Part model, mm, in its own coordinate system. Coordinates: 2 decimals unless noted, no trailing zeros. Write each loop counter-clockwise with the first axis right and the second up, starting at its lowest first coordinate (ties: lowest second). Pieces come first, ordered by that corner, then holes. Notation, with made-up numbers: (80.5, 25.25) -> (125.5, 25.25) arc R32 cw to (125.5, 60.25) -> close; hole circle Ø3 at (51, -16.75). An arc over 180 degrees is marked (long way). Write item = value, one per line.
Autodesk Inventor part; units mm, degrees
ref_plane "YZ Plane" through (0, 0, 0) normal (1, 0, 0) x (0, 1, 0)
ref_plane "XZ Plane" through (0, 0, 0) normal (0, 1, 0) x (-1, 0, 0)
ref_plane "XY Plane" through (0, 0, 0) normal (0, 0, 1) x (1, 0, 0)
sketch "スケッチ1" plane through (0, 0, 0) normal (0, 0, 1) x (1, 0, 0)
  circle A0 centre (-5, 0) radius 1.55
  line L0 (0, 0) -> (-5, 0) construction
  line L1 (0, 0) -> (5, 0) construction
  circle A1 centre (5, 0) radius 1.55
  line L2 (-5, 3) -> (5, 3)
  arc A2 (-5, 3) -> (-5, -3) centre (-5, 0) ccw
  line L3 (-5, -3) -> (5, -3)
  arc A3 (5, -3) -> (5, 3) centre (5, 0) ccw
  dimension "d0" = 5
  dimension "d1" = 3.1
  dimension "d2" = 3
extrude "押し出し1" add sketch "スケッチ1" along normal blind 8
properties part number "胴体_サブフレーム_1_8" material "アセタール樹脂、黒"
Q1. Probe line 1 (X direction, y = -0.5, z = 4.5); line 2 (Y direction, x = 5, z = 3.25); line 3 (X direction, y = 0.95, z = 4.5). List the from-to ranges inside material, lowest first. Write a range as from..to.
Model answer:
line_1 = -7.96..-6.47, -3.53..3.53, 6.47..7.96
line_2 = -3..-1.55, 1.55..3
line_3 = -7.85..-6.22, -3.78..3.78, 6.22..7.85
Q2. Mould opens along X. For faces 1 (the face through (0, 0, 8)), 2 (the face through (8, 0, 4)), 3 (the face through (3.45, -0.07, 3.94)) say: released by +X, released by -X, zero draft, split by the parting line, or undercut.
Model answer:
face_1 = zero draft
face_2 = released by +X
face_3 = undercut
Q3. Saw through at C-C on x = 5.75. Give the cut face in (y, z).
Model answer:
outline = (-2.9, 0) -> (-1.36, 0) -> (-1.36, 8) -> (-2.9, 8) -> close; (1.36, 0) -> (2.9, 0) -> (2.9, 8) -> (1.36, 8) -> close
Q4. Saw through at A-A on y = 0. Give the cut face in (x, z).
Model answer:
outline = (-8, 0) -> (-6.55, 0) -> (-6.55, 8) -> (-8, 8) -> close; (-3.45, 0) -> (3.45, 0) -> (3.45, 8) -> (-3.45, 8) -> close; (6.55, 0) -> (8, 0) -> (8, 8) -> (6.55, 8) -> close
Q5. Pin check, flat tip, straight feed: pin 1 (3 mm diameter, centred on y = 2, z = 5.5, fed in from -X). Stop position of the tip, or through.
Model answer:
pin_1 = -7.96
Q6. Saw through at B-B on z = 1.25. Give the cut face in (x, y).
Model answer:
outline = (-5, -3) -> (5, -3) arc R3 ccw to (5, 3) -> (-5, 3) arc R3 ccw to start; hole circle Ø3.1 at (-5, 0); hole circle Ø3.1 at (5, 0)
